Input: part model. Units: mm. Frame: model coordinates. Face numbers are marked on the shaded views. A direction names the side the tool comes from. Give positions to 0.01 mm unless a question says otherwise; leave off trailing zeros. Order: outer loops, then holes, each group sorted by start corner. A loop starts at its lowest first (then second) coordinate and runs counter-clockwise, first axis right, second up. Notation, with made-up numbers: (33, -26) - (72, -26) arc R25 cw to (72, 3) - close; hole circle Ø10 at (81, 54.5). An arc over 180 degrees is marked (long way). Use a Markdown table: item, result.
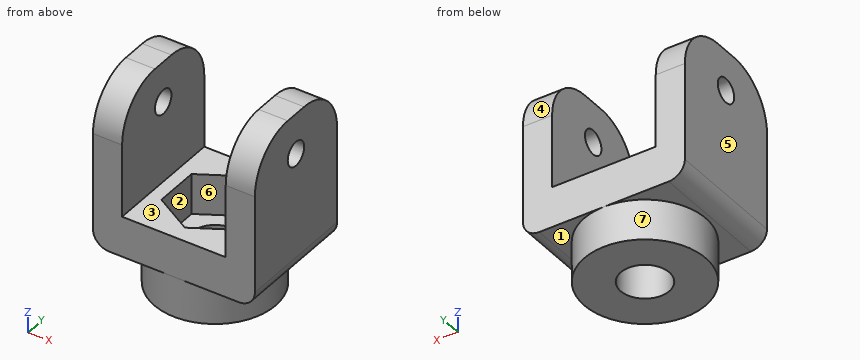
from build123d import *

# Parameters (mm, degrees)
SKETCH_R     = 7.5
SKETCH_R_2   = 3
PAD_DEPTH    = 5
SKETCH001_W  = 20
SKETCH001_H  = 15
PAD001_DEPTH = 5
SKETCH002_W  = 3.6
SKETCH002_H  = 15
PAD002_DEPTH = 15
SKETCH003_R  = 1.5
POCKET_DEPTH = 20.001
FILLET_R     = 2
FILLET001_R  = 6


with BuildPart() as part:
    # Sketch → Pad (new body)
    with BuildSketch(Plane.XY):
        Circle(SKETCH_R)
        Circle(SKETCH_R_2, mode=Mode.SUBTRACT)
    extrude(amount=PAD_DEPTH)

    # Sketch001 (on Face4 of Pad) → Pad001 (join)
    with BuildSketch(Plane.XY.offset(5)):
        Rectangle(SKETCH001_W, SKETCH001_H)
        Polygon((4.76314, -2.75), (4.76314, 2.75), (0, 5.5), (-4.76314, 2.75), (-4.76314, -2.75), (0, -5.5), align=None, mode=Mode.SUBTRACT)
    extrude(amount=PAD001_DEPTH)

    # Sketch002 (on Face11 of Pad001) → Pad002 (join)
    with BuildSketch(Plane.XY.offset(10)):
        with Locations((-8.2, 0)):
            Rectangle(SKETCH002_W, SKETCH002_H)
        with Locations((8.2, 0)):
            Rectangle(SKETCH002_W, SKETCH002_H)
    extrude(amount=PAD002_DEPTH)

    # Sketch003 (on Face17 of Pad002) → Pocket (cut, through all)
    with BuildSketch(Plane(origin=(-10, 0, 0), x_dir=(0, -1, 0), z_dir=(-1, 0, 0))):
        with Locations((0, 20)):
            Circle(SKETCH003_R)
    extrude(amount=-POCKET_DEPTH, mode=Mode.SUBTRACT)

    # Fillet
    fillet_edges = [part.edges().sort_by_distance(p)[0] for p in [
        (-10, 0, 5),
        (10, 0, 5),
    ]]
    fillet(fillet_edges, radius=FILLET_R)

    # Fillet001
    fillet001_edges = [part.edges().sort_by_distance(p)[0] for p in [
        (-8.2, -7.5, 25),
        (-8.2, 7.5, 25),
        (8.2, 7.5, 25),
        (8.2, -7.5, 25),
    ]]
    fillet(fillet001_edges, radius=FILLET001_R)


solid = part.part
1. Mould query, pull axis Y, two halves, no side actions, for the marked faces 4, 5, 6 and 7. Classes: pulls with the +Y half, pulls with the -Y half, needs draft (parallel to the pull), parting line crosses it, or undercut.
Response:
| item | result |
|---|---|
| face 4 | pulls with the +Y half |
| face 5 | needs draft |
| face 6 | undercut |
| face 7 | parting line crosses it |
2. Section query D-D (z = 9.25). Return loops of the section in (x, y), then the cut area to 3 significant figures.
Response:
| item | result |
|---|---|
| outline | (-10, -7.5) - (10, -7.5) - (10, 7.5) - (-10, 7.5) - close; hole (-4.76, -2.75) - (0, -5.5) - (4.76, -2.75) - (4.76, 2.75) - (0, 5.5) - (-4.76, 2.75) - close |
| area | 221 mm^2 |
3. Section query B-B (z = 12.5). Return loops of the section in (x, y).
Response:
| item | result |
|---|---|
| outline | (-10, -7.5) - (-6.4, -7.5) - (-6.4, 7.5) - (-10, 7.5) - close; (6.4, -7.5) - (10, -7.5) - (10, 7.5) - (6.4, 7.5) - close |
4. Section query A-A (y = 0). State how many separate pieces and enclosed holes the cut face has, then the cut area to 3 significant figures.
Response:
| item | result |
|---|---|
| separate pieces | 4 |
| enclosed holes | 0 |
| area | 182 mm^2 |
5. Pin query (flat end, axial travel): pin 1 (3 mm diameter, centred on x = 7, y = 4, fed in from +Z); pin 2 (1.8 mm diameter, centred on y = 0, z = 20, fed in from -X); pin 3 (7.5 mm diameter, centred on x = 1.5, y = 0, fed in from +Z); pin 4 (2 mm diameter, centred on x = -7.5, y = 4.5, fed in from -Z). Return the tip coordinate at first contact, or that it passes through.
Response:
| item | result |
|---|---|
| pin 1 | stops at z = 24.92 |
| pin 2 | passes through |
| pin 3 | stops at z = 10 |
| pin 4 | stops at z = 5 |
6. Set-up query: the marked faces 1, 2 and 3. Return all of +Z, -Z, +X, -X, +Y, -Y with unobstructed straight access to the full face (end or side cutting, diameter ignored); none if empty.
Response:
| item | result |
|---|---|
| face 1 | -Z, +X |
| face 2 | +Z |
| face 3 | +Z, +Y, -Y |
7. Material intervals for line 1 along Z through (x, y) = (8.05, 0); line 2 along X through (y, z) = (6.5, 19.5); line 3 along Y through (x, z) = (0, 2.3), sorted ascending.
Response:
| item | result |
|---|---|
| line 1 | z = 5 to 18.5, 21.5 to 25 |
| line 2 | x = -10 to -6.4, 6.4 to 10 |
| line 3 | y = -7.5 to -3, 3 to 7.5 |
8. Section query C-C (x = -6). Return loops of the section in (y, z).
Response:
| item | result |
|---|---|
| outline | (-7.5, 5) - (-4.5, 5) - (-4.5, 0) - (4.5, 0) - (4.5, 5) - (7.5, 5) - (7.5, 10) - (-7.5, 10) - close |
